Part model, mm, in its own coordinate system. A direction names the side the tool comes from. Give positions to 0.01 mm unless a question says otherwise; leave off trailing zeros. Order: outer loops, then holes, each group sorted by start corner. A loop starts at its lowest first (then second) coordinate and runs counter-clockwise, first axis right, second up. Notation, with made-up numbers: (52, 24) -> (76, 24) arc R20 cw to (76, 42) -> close; hole circle Ø11 at (26, 42). An arc over 180 degrees is marked (long way). Write item = value, one per line. Start each with the question number.
(1) Saw through at C-C, the plane x = -0.5. List the corners of the cut face in (y, z), then the cut area to 3 significant figures.
(2) Probe line 1 along Y through (x, z) = (0, 3.25); line 2 along Y through (x, z) = (0, 15.25); line 3 along Y through (x, z) = (0, 9.75). List the from-to ranges inside material, lowest first. Write a range as from..to.
(3) Two-plate mould, pull along Y, no slides. Class faces 3 (the flat face through (0, -40, 10)), 4 (the cylindrical face through (-4.05, 28.72, 16.84)), 5 (the flat face through (7.5, -1, 5)): pulls with the +Y half, pulls with the -Y half, needs draft (parallel to the pull), parting line crosses it, or undercut.
(4) Saw through at D-D, the plane z = 18. List the corners of the cut face in (x, y).
(5) Flat gauge pin, fed straight in: pin 1 (3.5 mm diameter, centred on x = 2, y = 22.5, fed in from +Z). Where does the tip first touch, or does it go through?
(6) Saw through at A-A, the plane y = 0. List the corners of the cut face in (x, z), then the cut area to 3 significant figures.
(7) Saw through at B-B, the plane z = 10. List the corners of the cut face in (x, y).
(8) Which spindle directions (+Z, -Z, +X, -X, +Y, -Y) get a long thin tool onto all of the face, cutting with end or side? Do faces 1 (the flat face through (0, 1, 0)), 2 (the flat face through (2.4, -27.4, 13.6)). Say none if no direction does.
from build123d import *

# Parameters (mm, degrees)
SKETCH_1_W                   = 15
SKETCH_1_H                   = 80
EXTRUDE_1_DEPTH              = 20
HOLE_WIZARD_M8_1_D           = 6.8
HOLE_WIZARD_M8_1_DEPTH       = 19.75
HOLE_WIZARD_M8_1_TIP         = 2.042926105
HOLE_WIZARD_M6_1_D           = 6.4
HOLE_WIZARD_M6_1_CBORE_D     = 11
HOLE_WIZARD_M6_1_CBORE_DEPTH = 6.4


with BuildPart() as part:
    # 草图1 → 凸台-拉伸1 (new body)
    with BuildSketch(Plane.XY):
        Rectangle(SKETCH_1_W, SKETCH_1_H)
    extrude(amount=EXTRUDE_1_DEPTH)

    # M8 螺纹孔1
    with Locations(Plane(origin=(7.5, 0, 10), x_dir=(0, 0, 1), z_dir=(1, 0, 0))):
        with Locations((0, 0)):
            Hole(HOLE_WIZARD_M8_1_D / 2, depth=HOLE_WIZARD_M8_1_DEPTH)
            with Locations((0, 0, -(HOLE_WIZARD_M8_1_DEPTH + HOLE_WIZARD_M8_1_TIP / 2))):  # 118° drill point
                Cone(0, HOLE_WIZARD_M8_1_D / 2, HOLE_WIZARD_M8_1_TIP, mode=Mode.SUBTRACT)

    # M6 六角凹头螺钉的柱形沉头孔1 (through all)
    with Locations(Plane(origin=(0, 25, 20), x_dir=(1, 0, 0), z_dir=(0, 0, 1))):
        with Locations((0, 0), (0, -50)):
            CounterBoreHole(HOLE_WIZARD_M6_1_D / 2, HOLE_WIZARD_M6_1_CBORE_D / 2, HOLE_WIZARD_M6_1_CBORE_DEPTH)


solid = part.part
Results list:
q1.outline = (-40, 0) -> (-28.16, 0) -> (-28.16, 13.6) -> (-30.48, 13.6) -> (-30.48, 20) -> (-40, 20) -> close; (-21.84, 0) -> (21.84, 0) -> (21.84, 13.6) -> (19.52, 13.6) -> (19.52, 20) -> (-19.52, 20) -> (-19.52, 13.6) -> (-21.84, 13.6) -> close; (28.16, 0) -> (40, 0) -> (40, 20) -> (30.48, 20) -> (30.48, 13.6) -> (28.16, 13.6) -> close; hole circle Ø6.8 at (0, 10)
q1.area = 1,250 mm^2
q2.line_1 = -40..-28.2, -21.8..21.8, 28.2..40
q2.line_2 = -40..-30.5, -19.5..19.5, 30.5..40
q2.line_3 = -40..-28.2, -21.8..-3.39, 3.39..21.8, 28.2..40
q3.face_3 = pulls with the -Y half
q3.face_4 = undercut
q3.face_5 = needs draft
q4.outline = (-7.5, -40) -> (7.5, -40) -> (7.5, 40) -> (-7.5, 40) -> close; hole circle Ø11 at (0, -25); hole circle Ø11 at (0, 25)
q5.pin_1 = 13.6
q6.outline = (-7.5, 0) -> (7.5, 0) -> (7.5, 6.6) -> (-7.5, 6.6) -> close; (-7.5, 13.4) -> (7.5, 13.4) -> (7.5, 20) -> (-7.5, 20) -> close
q6.area = 198 mm^2
q7.outline = (-7.5, -40) -> (7.5, -40) -> (7.5, -3.4) -> (-7.5, -3.4) -> close; (-7.5, 3.4) -> (7.5, 3.4) -> (7.5, 40) -> (-7.5, 40) -> close; hole circle Ø6.4 at (0, -25); hole circle Ø6.4 at (0, 25)
q8.face_1 = -Z, +X, -X, +Y, -Y
q8.face_2 = +Z
